Input: part model. Units: mm. Frame: model coordinates. A direction names the side the tool comes from. Give positions to 0.01 mm unless a question says otherwise; leave off trailing zeros. Loops run counter-clockwise (first coordinate to the right, second up) from the corner with the lowest first, then second, coordinate; pieces in that order, holes last. Notation, with made-up numbers: (48.5, -15.75) - (67.5, -15.75) arc R31 ccw to (67.5, 17.25) - close; hole circle Ø10 at (84.5, 57.25). An arc over 180 degrees is marked (long way). Answer as a JSON object with one key per item and string values.
from build123d import *

# Parameters (mm, degrees)
SKETCH1_W           = 61.05
SKETCH1_H           = 45
BOSS_EXTRUDE2_DEPTH = 5
SKETCH2_W           = 10
SKETCH2_H           = 10
BOSS_EXTRUDE3_DEPTH = 22.5
SKETCH3_R           = 4
CUT_EXTRUDE1_DEPTH  = 8
SKETCH6_W           = 15
SKETCH6_H           = 30
BOSS_EXTRUDE4_DEPTH = 30
SKETCH7_W           = 15
SKETCH7_H           = 17
CUT_EXTRUDE3_DEPTH  = 23
SKETCH8_R           = 2.5
CUT_EXTRUDE4_DEPTH  = 84.529051832
SKETCH9_W           = 5
SKETCH9_H           = 45
BOSS_EXTRUDE5_DEPTH = 68
SKETCH10_R          = 2.5
CUT_EXTRUDE5_DEPTH  = 5
CUT_EXTRUDE6_DEPTH  = 16


with BuildPart() as part:
    # Sketch1 → Boss-Extrude2 (new body)
    with BuildSketch(Plane(origin=(0, 0, 0), x_dir=(1, 0, 0), z_dir=(0, 1, 0))):
        with Locations((30.525, 22.5)):
            Rectangle(SKETCH1_W, SKETCH1_H)
    extrude(amount=BOSS_EXTRUDE2_DEPTH)

    # Sketch2 → Boss-Extrude3 (add)
    with BuildSketch(Plane(origin=(0, 5, 0), x_dir=(1, 0, 0), z_dir=(0, 1, 0))):
        with Locations((20, 35)):
            Rectangle(SKETCH2_W, SKETCH2_H)
    extrude(amount=BOSS_EXTRUDE3_DEPTH)

    # Sketch3 → Cut-Extrude1 (cut)
    with BuildSketch(Plane(origin=(0, 0, -40), x_dir=(-1, 0, 0), z_dir=(0, 0, -1))):
        with Locations((-20, 20.9)):
            Circle(SKETCH3_R)
    extrude(amount=-CUT_EXTRUDE1_DEPTH, mode=Mode.SUBTRACT)

    # Sketch6 → Boss-Extrude4 (add)
    with BuildSketch(Plane(origin=(0, 5, 0), x_dir=(1, 0, 0), z_dir=(0, 1, 0))):
        with Locations((20, 15)):
            Rectangle(SKETCH6_W, SKETCH6_H)
    extrude(amount=BOSS_EXTRUDE4_DEPTH)

    # Sketch7 → Cut-Extrude3 (cut)
    with BuildSketch(Plane.XY):
        with Locations((20, 21.7)):
            Rectangle(SKETCH7_W, SKETCH7_H)
    extrude(amount=-CUT_EXTRUDE3_DEPTH, mode=Mode.SUBTRACT)

    # Sketch8 → Cut-Extrude4 (cut, through all)
    with BuildSketch(Plane(origin=(0, 35, 0), x_dir=(1, 0, 0), z_dir=(0, 1, 0))):
        with Locations(Location((20, 7.5, 0), (0, 0, 270))):
            Circle(SKETCH8_R)
    extrude(amount=-CUT_EXTRUDE4_DEPTH, mode=Mode.SUBTRACT)

    # Sketch9 → Boss-Extrude5 (add)
    with BuildSketch(Plane.XZ):
        with Locations((58.55, -22.5)):
            Rectangle(SKETCH9_W, SKETCH9_H)
    extrude(amount=BOSS_EXTRUDE5_DEPTH)

    # Sketch10 → Cut-Extrude5 (cut)
    with BuildSketch(Plane(origin=(61.05, 0, 0), x_dir=(0, 0, -1), z_dir=(1, 0, 0))):
        with Locations((13.274189438, -45)):
            Circle(SKETCH10_R)
        with Locations((33.274189438, -45)):
            Circle(SKETCH10_R)
    extrude(amount=-CUT_EXTRUDE5_DEPTH, mode=Mode.SUBTRACT)

    # Sketch11 → Cut-Extrude6 (cut)
    with BuildSketch(Plane.XY):
        Polygon((24.979172019, 9.2), (14.879172019, 9.2), (14.879172019, 7.5), (16.429172019, 7.5), (16.429172019, -2.944116306), (23.429172019, -2.944116306), (23.429172019, 7.5), (24.979172019, 7.5), align=None)
    extrude(amount=-CUT_EXTRUDE6_DEPTH, mode=Mode.SUBTRACT)


solid = part.part
Item 1: Cut plane C-C (y = -45). Return loops of the section in (x, z), then the cut area to 3 significant figures.
Geometry check:
{"outline": "(56.05, -45) - (61.05, -45) - (61.05, -35.77) - (56.05, -35.77) - close; (56.05, -30.77) - (61.05, -30.77) - (61.05, -15.77) - (56.05, -15.77) - close; (56.05, -10.77) - (61.05, -10.77) - (61.05, 0) - (56.05, 0) - close", "area": "175 mm2"}
Item 2: Access query for faces 4 (the face through (12.5, 13, -18)), 5 (the face through (28, 0, -23)), 6 (the face through (20, 30.2, -11)). Directions: +Z, -Z, +X, -X, +Y, -Y. A direction counts if a zero-diameter tool reaches every point of the face in a straight line with its end or side. Return the directions, or none.
Geometry check:
{"face 4": "+Z, -Z, -X, +Y", "face 5": "+Z, -Z, -X, -Y", "face 6": "+Z, +X, -X"}
Item 3: Cut plane D-D (z = -13.5). Return loops of the section in (x, y), then the cut area to 3 significant figures.
Geometry check:
{"outline": "(0, 0) - (16.43, 0) - (16.43, 7.5) - (14.88, 7.5) - (14.88, 9.2) - (24.98, 9.2) - (24.98, 7.5) - (23.43, 7.5) - (23.43, 0) - (56.05, 0) - (56.05, -42.51) - (61.05, -42.51) - (61.05, 5) - (27.5, 5) - (27.5, 13.2) - (12.5, 13.2) - (12.5, 5) - (0, 5) - close; (12.5, 30.2) - (27.5, 30.2) - (27.5, 35) - (12.5, 35) - close; (56.05, -68) - (61.05, -68) - (61.05, -47.49) - (56.05, -47.49) - close", "area": "746 mm2"}
Item 4: Cut plane B-B (x = 20). Return loops of the section in (y, z), then the cut area to 3 significant figures.
Geometry check:
{"outline": "(0, -45) - (5, -45) - (5, -40) - (16.9, -40) - (16.9, -32) - (24.9, -32) - (24.9, -40) - (27.5, -40) - (27.5, -30) - (35, -30) - (35, -10) - (30.2, -10) - (30.2, -23) - (13.2, -23) - (13.2, -10) - (9.2, -10) - (9.2, -16) - (0, -16) - close; (9.2, -5) - (13.2, -5) - (13.2, 0) - (9.2, 0) - close; (30.2, -5) - (35, -5) - (35, 0) - (30.2, 0) - close", "area": "704 mm2"}
Item 5: Cut plane A-A (z = -7.5). Give the number of separate pieces and of enclosed holes in the cut face, then the cut area to 3 significant figures.
Geometry check:
{"separate pieces": "4", "enclosed holes": "0", "area": "727 mm2"}
Item 6: Contact query for flat-ended pins moving along their axis: P1, Ø4, axis at y = 4.5, z = -5.5, coming from the -X side; P2, Ø4, axis at x = 20, y = 20, coming from the +Z side; P3, Ø5, axis at x = 22.5, z = -37.5, coming from the +Y side; P4, Ø3, axis at y = 17.5, z = -32.5, coming from the -X side. Output: stop coordinate, or through.
Geometry check:
{"P1": "stops at x = 0", "P2": "stops at z = -23", "P3": "stops at y = 27.5", "P4": "stops at x = 15"}
Item 7: Material intervals for line 1 (Y direction, x = 20, z = -38); line 2 (Y direction, x = 13, z = -18); line 3 (Y direction, x = 7.5, z = -20.5), sorted ascending. Write a range as [from, to].
Geometry check:
{"line 1": "y = [0, 16.9], [24.9, 27.5]", "line 2": "y = [0, 13.2], [30.2, 35]", "line 3": "y = [0, 5]"}
Item 8: Mould query, pull axis Y, two halves, no side actions, for faces 1 (the face through (15, 16, -35)), 2 (the face through (20, 27.5, -35)), 3 (the face through (20, 21, -32)). Classes: released by +Y, released by -Y, zero draft, split by the parting line, or undercut.
Geometry check:
{"face 1": "zero draft", "face 2": "released by +Y", "face 3": "undercut"}
